```python
from build123d import *

# Parameters (mm, degrees)
SKETCH1_R           = 60
SKETCH1_R_2         = 2
SKETCH1_R_3         = 4
SKETCH1_R_4         = 1.5
BOSS_EXTRUDE1_DEPTH = 1.5


with BuildPart() as part:
    # Sketch1 → Boss-Extrude1 (new body)
    with BuildSketch(Plane(origin=(0, 0, 0), x_dir=(1, 0, 0), z_dir=(0, 1, 0))):
        with Locations(Location((0, 0, 0), (0, 0, 270))):
            Circle(SKETCH1_R)
        with Locations(Location((0, 49.5, 0), (0, 0, 270))):
            Circle(SKETCH1_R_2, mode=Mode.SUBTRACT)
        with Locations(Location((-49.5, 0, 0), (0, 0, 270))):
            Circle(SKETCH1_R_2, mode=Mode.SUBTRACT)
        with Locations(Location((0, -49.5, 0), (0, 0, 270))):
            Circle(SKETCH1_R_2, mode=Mode.SUBTRACT)
        with Locations(Location((49.5, 0, 0), (0, 0, 270))):
            Circle(SKETCH1_R_2, mode=Mode.SUBTRACT)
        with Locations(Location((0, 35, 0), (0, 0, 270))):
            Circle(SKETCH1_R_3, mode=Mode.SUBTRACT)
        with Locations(Location((0, 41.9, 0), (0, 0, 270))):
            Circle(SKETCH1_R_4, mode=Mode.SUBTRACT)
        with Locations(Location((6.9, 35, 0), (0, 0, 270))):
            Circle(SKETCH1_R_4, mode=Mode.SUBTRACT)
        with Locations(Location((0, 28.1, 0), (0, 0, 270))):
            Circle(SKETCH1_R_4, mode=Mode.SUBTRACT)
        with Locations(Location((-6.9, 35, 0), (0, 0, 270))):
            Circle(SKETCH1_R_4, mode=Mode.SUBTRACT)
        with Locations(Location((0, -35, 0), (0, 0, 90))):
            Circle(SKETCH1_R_3, mode=Mode.SUBTRACT)
        with Locations(Location((0, -28.1, 0), (0, 0, 90))):
            Circle(SKETCH1_R_4, mode=Mode.SUBTRACT)
        with Locations(Location((-6.9, -35, 0), (0, 0, 90))):
            Circle(SKETCH1_R_4, mode=Mode.SUBTRACT)
        with Locations(Location((0, -41.9, 0), (0, 0, 90))):
            Circle(SKETCH1_R_4, mode=Mode.SUBTRACT)
        with Locations(Location((6.9, -35, 0), (0, 0, 90))):
            Circle(SKETCH1_R_4, mode=Mode.SUBTRACT)
        with Locations(Location((-34.2, 5, 0), (0, 0, 270))):
            Circle(SKETCH1_R_2, mode=Mode.SUBTRACT)
        with Locations(Location((-34.2, -5, 0), (0, 0, 90))):
            Circle(SKETCH1_R_2, mode=Mode.SUBTRACT)
        with Locations(Location((14.2, 5, 0), (0, 0, 90))):
            Circle(SKETCH1_R_2, mode=Mode.SUBTRACT)
        with Locations(Location((14.2, -5, 0), (0, 0, 270))):
            Circle(SKETCH1_R_2, mode=Mode.SUBTRACT)
        with BuildLine():
            Line((-37.5, -1.5), (-30.5, -1.5))
            Line((-30.5, -1.5), (-30.5, -10))
            ThreePointArc((-30.5, -10), (-30.353553391, -10.353553391), (-30, -10.5))
            Line((-30, -10.5), (10, -10.5))
            ThreePointArc((10, -10.5), (10.353553391, -10.353553391), (10.5, -10))
            Line((10.5, -10), (10.5, -1.5))
            Line((10.5, -1.5), (17.5, -1.5))
            ThreePointArc((17.5, -1.5), (19, 0), (17.5, 1.5))
            Line((17.5, 1.5), (10.5, 1.5))
            Line((10.5, 1.5), (10.5, 10))
            ThreePointArc((10.5, 10), (10.353553391, 10.353553391), (10, 10.5))
            Line((10, 10.5), (-30, 10.5))
            ThreePointArc((-30, 10.5), (-30.353553391, 10.353553391), (-30.5, 10))
            Line((-30.5, 10), (-30.5, 1.5))
            Line((-30.5, 1.5), (-37.5, 1.5))
            ThreePointArc((-37.5, 1.5), (-39, 0), (-37.5, -1.5))
        make_face(mode=Mode.SUBTRACT)
    extrude(amount=BOSS_EXTRUDE1_DEPTH)


solid = part.part
```
Part model, mm, in its own coordinate system. Coordinates: 2 decimals unless noted, no trailing zeros. Write each loop counter-clockwise with the first axis right and the second up, starting at its lowest first coordinate (ties: lowest second). Pieces come first, ordered by that corner, then holes.
Item 1: Mould opens along Z. For faces 1 (the face through (2.64, 0.74, -59.94)), 2 (the face through (47.726, 0.74, 0.923)), 3 (the face through (1, 0, 12)) say: released by +Z, released by -Z, zero draft, split by the parting line, or undercut.
Item 2: Slice it at D-D (x = 49.5). Write the cut outline in (y, z), and give its area (3 significant figures).
Item 3: Pin check, flat tips, straight feed: pin 1 (3 mm diameter, centred on x = 0, z = -49.5, fed in from +Y); pin 2 (0.8 mm diameter, centred on x = -3.5, y = 1, fed in from -Z). Stop position of each tip, or through.
Item 4: Slice it at B-B (z = 35). Write the cut outline in (x, y).
Item 5: Slice it at A-A (x = 6.9). Write the cut outline in (y, z).
Item 6: Probe line 1 (Z direction, x = -8, y = 0.85); line 2 (X direction, y = 1.1, z = -35); line 3 (X direction, y = 0.9, z = 5). List the from-to ranges inside material, lowest first.
Item 7: Slice it at C-C (z = 49.5). Write the cut outline in (x, y), and give its area (3 significant figures).
Results found:
1. face 1: split by the parting line
1. face 2: undercut
1. face 3: zero draft
2. outline: (0, -33.91) - (1.5, -33.91) - (1.5, -2) - (0, -2) - close; (0, 2) - (1.5, 2) - (1.5, 33.91) - (0, 33.91) - close
2. area: 95.7 mm2
3. pin 1: passes through
3. pin 2: stops at z = -59.92
4. outline: (-48.73, 0) - (-8.4, 0) - (-8.4, 1.5) - (-48.73, 1.5) - close; (-5.4, 0) - (-4, 0) - (-4, 1.5) - (-5.4, 1.5) - close; (4, 0) - (5.4, 0) - (5.4, 1.5) - (4, 1.5) - close; (8.4, 0) - (48.73, 0) - (48.73, 1.5) - (8.4, 1.5) - close
5. outline: (0, -59.6) - (1.5, -59.6) - (1.5, -36.5) - (0, -36.5) - close; (0, -33.5) - (1.5, -33.5) - (1.5, -10.5) - (0, -10.5) - close; (0, 10.5) - (1.5, 10.5) - (1.5, 33.5) - (0, 33.5) - close; (0, 36.5) - (1.5, 36.5) - (1.5, 59.6) - (0, 59.6) - close
6. line 1: z = -59.46 to -36.02, -33.98 to -10.5, 10.5 to 33.98, 36.02 to 59.46
6. line 2: x = -48.73 to -8.4, -5.4 to -4, 4 to 5.4, 8.4 to 48.73
6. line 3: x = -59.79 to -36.2, -32.2 to -30.5, 10.5 to 12.2, 16.2 to 59.79
7. outline: (-33.91, 0) - (-2, 0) - (-2, 1.5) - (-33.91, 1.5) - close; (2, 0) - (33.91, 0) - (33.91, 1.5) - (2, 1.5) - close
7. area: 95.7 mm2
